```python
from build123d import *

# Parameters (mm, degrees)
F0_W     = 37.331247
F0_H     = 27.314525
F1_DEPTH = 25.4
F3_DEPTH = 26.944021


with BuildPart() as f1:
    # F0 (on Top) → F1 (new body)
    with BuildSketch(Plane.XY):
        Polygon((-5.064317, -18.266939), (-41.957065, -18.266939), (-41.957065, -53.090654), (-5.064317, -53.090654), (-5.064317, -45.581464), align=None)
        with Locations((13.601306, -31.924201)):
            Rectangle(F0_W, F0_H)
    extrude(amount=F1_DEPTH)

    # F2 (on face) → F3 (join)
    with BuildSketch(Plane.XY.offset(25.4)):
        Polygon((30.699346, -20.429492), (-39.95049, -21.168509), (-39.95049, -50.943833), (-39.442882, -50.934415), (-6.923128, -51.261608), (-6.923128, -44.098966), (30.813994, -44.266075), (30.813994, -20.261256), align=None)
    extrude(amount=F3_DEPTH)


solid = f1.part
```
Here's how the part is built. I have some questions about the finished solid (model axes, mm). A direction names the side the tool comes from. Round coordinates to 2 decimals unless told otherwise and drop trailing zeros. Loops run counter-clockwise (first coordinate to the right, second up) from the corner with the lowest first, then second, coordinate; pieces in that order, holes last.
1. Suppose I cut it at B-B, the plane z = 46. Please give me the cut outline in (x, y), and give its area (3 significant figures).
Answers:
outline: (-39.95, -50.94) - (-39.44, -50.93) - (-6.92, -51.26) - (-6.92, -44.1) - (30.81, -44.27) - (30.81, -20.26) - (30.7, -20.43) - (-39.95, -21.17) - close
area: 1,880 mm2
2. For faces 1 (the face through (30.814, -32, 39)), 2 (the face through (-39.95, -36, 39)), 3 (the face through (-24, -53.091, 13)), 4 (the face through (13, -45.581, 13)), which set-ups out of +Z, -Z, +X, -X, +Y, -Y let a thin tool reach every point of the face, with its end or its side?
Answers:
face 1: +Z, +X, +Y, -Y
face 2: +Z, -X, +Y, -Y
face 3: +Z, -Z, +X, -X, -Y
face 4: +Z, -Z, +X, -Y
3. Will these pins go through, and if not, where does the flat tip stop? pin 1 (4 mm diameter, centred on y = -50, z = 18.5, fed in from +X); pin 2 (5 mm diameter, centred on x = 5, z = 26.5, fed in from -Y); pin 3 (19 mm diameter, centred on y = -28, z = 43.5, fed in from +X).
Answers:
pin 1: stops at x = -5.06
pin 2: stops at y = -45.58
pin 3: stops at x = 30.81
4. If I drill on probe 1 along X at (y, z) = (-45.5, 35); probe 2 along Y at (x, z) = (9, 14.5); probe 3 along X at (y, z) = (-35, 36), over which ranges is the centre line in solid material (lowest first)?
Answers:
probe 1: x = -39.95 to -6.92
probe 2: y = -45.58 to -18.27
probe 3: x = -39.95 to 30.81
5. Suppose I cut it at A-A, the plane y = -26. Please give me the cut outline in (x, z), and give its area (3 significant figures).
Answers:
outline: (-41.96, 0) - (32.27, 0) - (32.27, 25.4) - (30.81, 25.4) - (30.81, 52.34) - (-39.95, 52.34) - (-39.95, 25.4) - (-41.96, 25.4) - close
area: 3,790 mm2
6. Suppose I cut it at C-C, the plane z = 17. Please give me the cut outline in (x, y), and give its area (3 significant figures).
Answers:
outline: (-41.96, -53.09) - (-5.06, -53.09) - (-5.06, -45.58) - (32.27, -45.58) - (32.27, -18.27) - (-41.96, -18.27) - close
area: 2,300 mm2
